Could you check a few things on this model? Use its own coordinates, in mm. A direction names the side the tool comes from. Coordinates: 2 decimals unless noted, no trailing zeros. Loops run counter-clockwise (first coordinate to the right, second up) from the corner with the lowest first, then second, coordinate; pieces in that order, holes last. Notation, with made-up numbers: (64.5, -38.5) - (73.5, -38.5) arc R11 ccw to (73.5, -17.5) - close; hole circle Ø9 at (-31, 2.5). An arc over 180 degrees is marked (long way). One line per question, with ' | ' between items. Start each with the question number.
1. We'd pull the mould along X, two halves only. Please class faces 1 (the flat face through (-111, 7, 0)), 2 (the flat face through (-62, 111, 52)): pulls with the +X half, pulls with the -X half, needs draft (parallel to the pull), parting line crosses it, or undercut.
2. I want a section at D-D, the plane z = 30. Count the separate pieces of the cut face and the enclosed holes in it, then the cut area to 3 significant figures.
3. I'm going to push flat-ended pins straight in: P1, Ø5, axis at y = 62.5, z = 41, coming from the -X side; P2, Ø3.5, axis at x = 10.5, y = 105.5, coming from the +Z side; P3, Ø6, axis at x = -11, y = 53.5, coming from the +Z side; P4, Ø1.5, axis at y = 60, z = 36, coming from the +X side. Where does each tip first touch, or does it pass through?
4. I want a section at B-B, the plane y = 59. Write out the boundary of the cut face in (x, z).
5. I want a section at C-C, the plane y = 74. Write out the boundary of the cut face in (x, z), then the cut area to 3 significant figures.
6. Which directions (+Z, -Z, +X, -X, +Y, -Y) give clear straight access to the entire face, cutting with the end or side of a thin tool? Please do faces 3 (the flat face through (281, 14, 7)), 4 (the flat face through (-115, 7, 10)), 5 (the flat face through (-111, 3, 11)), 6 (the flat face through (147, 106, 34)).
7. Please list where these lines run through material, in increasing order: L1, parallel to X at y = 59, z = 53; L2, parallel to Y at x = -59, z = 54; L3, parallel to X at y = 70.5, z = 9.5. Write a range as [from, to].
8. I want a section at A-A, the plane x = -59. Write out the boundary of the cut face in (y, z).
from build123d import *

# Parameters (mm, degrees)
F0_W      = 118
F0_H      = 118
F1_DEPTH  = 55
F3_DEPTH  = 3
F4_R      = 51.5
F5_DEPTH  = 100
F7_DEPTH  = 150
F9_DEPTH  = 111
F11_DEPTH = 290
F12_W     = 283
F12_H     = 86
F13_DEPTH = 50
F15_DEPTH = 150
F17_DEPTH = 25


with BuildPart() as f1:
    # F0 (on Top) → F1 (new body)
    with BuildSketch(Plane.XY):
        with Locations((-59, 59)):
            Rectangle(F0_W, F0_H)
    extrude(amount=F1_DEPTH)

    # F2 (on face) → F3 (cut)
    with BuildSketch(Plane.XY.offset(55)):
        with BuildLine():
            Line((-59, 59), (-5.5, 59))
            ThreePointArc((-5.5, 59), (-5.565833, 61.653265), (-5.763171, 64.3))
            ThreePointArc((-5.763171, 64.3), (-96.830213, 96.830213), (-64.3, 5.763171))
            ThreePointArc((-64.3, 5.763171), (-61.653265, 5.565833), (-59, 5.5))
            Line((-59, 5.5), (-59, 59))
        make_face()
        with BuildLine():
            ThreePointArc((-59, 5.5), (-61.653265, 5.565833), (-64.3, 5.763171))
            Line((-64.3, 5.763171), (-64.3, 2.463171))
            Line((-64.3, 2.463171), (-53.7, 2.463171))
            Line((-53.7, 2.463171), (-53.7, 5.763171))
            ThreePointArc((-53.7, 5.763171), (-56.346735, 5.565833), (-59, 5.5))
        make_face()
        with BuildLine():
            Line((-21.169787, 21.169787), (-59, 59))
            Line((-59, 59), (-59, 5.5))
            ThreePointArc((-59, 5.5), (-56.346735, 5.565833), (-53.7, 5.763171))
            ThreePointArc((-53.7, 5.763171), (-38.526436, 9.572445), (-25.103543, 17.608211))
            ThreePointArc((-25.103543, 17.608211), (-23.09248, 19.340197), (-21.169787, 21.169787))
        make_face()
        with BuildLine():
            Line((-15.274759, 22.770091), (-17.608211, 25.103543))
            ThreePointArc((-17.608211, 25.103543), (-19.340197, 23.09248), (-21.169787, 21.169787))
            ThreePointArc((-21.169787, 21.169787), (-23.09248, 19.340197), (-25.103543, 17.608211))
            Line((-25.103543, 17.608211), (-22.770091, 15.274759))
            Line((-22.770091, 15.274759), (-15.274759, 22.770091))
        make_face()
        with BuildLine():
            ThreePointArc((-5.763171, 53.7), (-5.565833, 56.346735), (-5.5, 59))
            Line((-5.5, 59), (-59, 59))
            Line((-59, 59), (-21.169787, 21.169787))
            ThreePointArc((-21.169787, 21.169787), (-19.340197, 23.09248), (-17.608211, 25.103543))
            ThreePointArc((-17.608211, 25.103543), (-9.572445, 38.526436), (-5.763171, 53.7))
        make_face()
        with BuildLine():
            ThreePointArc((-5.763171, 64.3), (-5.565833, 61.653265), (-5.5, 59))
            ThreePointArc((-5.5, 59), (-5.565833, 56.346735), (-5.763171, 53.7))
            Line((-5.763171, 53.7), (-2.463171, 53.7))
            Line((-2.463171, 53.7), (-2.463171, 64.3))
            Line((-2.463171, 64.3), (-5.763171, 64.3))
        make_face()
    extrude(amount=-F3_DEPTH, mode=Mode.SUBTRACT)

    # F4 (on face) → F5 (cut)
    with BuildSketch(Plane.XY.offset(52)):
        with Locations((-59, 59)):
            Circle(F4_R)
    extrude(amount=-F5_DEPTH, mode=Mode.SUBTRACT)

    # F6 (on face) → F7 (cut)
    with BuildSketch(Plane.XZ):
        Polygon((-104, 7), (-104, 0), (-14, 0), (-14, 7), (-7, 7), (-7, 14), (-27, 48), (-91, 48), (-111, 14), (-111, 7), align=None)
    extrude(amount=-F7_DEPTH, mode=Mode.SUBTRACT)

    # F8 (on face) → F9 (cut)
    with BuildSketch(Plane(origin=(-118, 0, 0), x_dir=(0, -1, 0), z_dir=(-1, 0, 0))):
        Polygon((-104, 7), (-104, 0), (-14, 0), (-14, 7), (-7, 7), (-7, 14), (-27, 48), (-91, 48), (-111, 14), (-111, 7), align=None)
    extrude(amount=-F9_DEPTH, mode=Mode.SUBTRACT)

    # F10 (on face) → F11 (join)
    with BuildSketch(Plane.YZ):
        with BuildLine():
            Line((7, 48), (7, 0))
            Line((7, 0), (111, 0))
            Line((111, 0), (111, 48))
            Line((111, 48), (109.381048, 48))
            ThreePointArc((109.381048, 48), (59, 12.5), (8.618952, 48))
            Line((8.618952, 48), (7, 48))
        make_face()
    extrude(amount=F11_DEPTH)

    # F12 (on face) → F13 (cut)
    with BuildSketch(Plane(origin=(0, 0, 0), x_dir=(1, 0, 0), z_dir=(0, 0, -1))):
        with Locations((141.5, -59)):
            Rectangle(F12_W, F12_H)
    extrude(amount=-F13_DEPTH, mode=Mode.SUBTRACT)

    # F14 (on face) → F15 (cut)
    with BuildSketch(Plane.XZ.offset(-7)):
        Polygon((14, 7), (14, 0), (276, 0), (276, 7), (283, 7), (283, 14), (263, 34), (27, 34), (7, 14), (7, 7), align=None)
    extrude(amount=-F15_DEPTH, mode=Mode.SUBTRACT)

    # F16 (on face) → F17 (cut)
    with BuildSketch(Plane.YZ.offset(290)):
        with BuildLine():
            ThreePointArc((104, 23.350264), (59, 4), (14, 23.350264))
            Line((14, 23.350264), (14, 7))
            Line((14, 7), (21, 7))
            Line((21, 7), (21, 0))
            Line((21, 0), (97, 0))
            Line((97, 0), (97, 7))
            Line((97, 7), (104, 7))
            Line((104, 7), (104, 23.350264))
        make_face()
    extrude(amount=-F17_DEPTH, mode=Mode.SUBTRACT)


solid = f1.part
Results are:
1) face 1: needs draft | face 2: undercut
2) separate pieces: 5 | enclosed holes: 0 | area: 2,550 mm2
3) P1: stops at x = -7 | P2: stops at z = 42.89 | P3: passes through | P4: stops at x = 0
4) outline: (-118, 48) - (-110.5, 48) - (-110.5, 52) - (-112.5, 52) - (-112.5, 55) - (-118, 55) - close; (-7.5, 48) - (-7, 48) - (-7, 0) - (0, 0) - (0, 55) - (-2.46, 55) - (-2.46, 52) - (-7.5, 52) - close; (283, 4) - (290, 4) - (290, 12.5) - (283, 12.5) - close
5) outline: (-118, 48) - (-108.27, 48) - (-108.27, 52) - (-110.35, 52) - (-110.35, 55) - (-118, 55) - close; (-9.73, 48) - (-7, 48) - (-7, 0) - (0, 0) - (0, 55) - (-7.65, 55) - (-7.65, 52) - (-9.73, 52) - close; (283, 5.84) - (290, 5.84) - (290, 14.65) - (283, 14.65) - close | area: 521 mm2
6) face 3: none | face 4: -X | face 5: +Y, -Y | face 6: -Z, +Y, -Y
7) L1: x = [-118, -112.5], [-2.46, 0] | L2: y = [0, 2.46], [112.5, 118] | L3: x = [-7, 0], [283, 290]
8) outline: (0, 48) - (7.5, 48) - (7.5, 52) - (2.46, 52) - (2.46, 55) - (0, 55) - close; (110.5, 48) - (118, 48) - (118, 55) - (112.5, 55) - (112.5, 52) - (110.5, 52) - close
